from build123d import *

# Parameters (mm, degrees)
SALIENTE_EXTRUIR1_DEPTH = 25
REDONDEO1_R             = 7
VACIADO1_T              = -3


with BuildPart() as part:
    # Croquis1 → Saliente-Extruir1 (new body)
    with BuildSketch(Plane.XY):
        with BuildLine():
            Line((-110, 65.5), (110, 65.5))
            ThreePointArc((110, 65.5), (122.727922061, 60.227922061), (128, 47.5))
            Line((128, 47.5), (128, -47.5))
            ThreePointArc((128, -47.5), (122.727922061, -60.227922061), (110, -65.5))
            Line((110, -65.5), (-110, -65.5))
            ThreePointArc((-110, -65.5), (-122.727922061, -60.227922061), (-128, -47.5))
            Line((-128, -47.5), (-128, 47.5))
            ThreePointArc((-128, 47.5), (-122.727922061, 60.227922061), (-110, 65.5))
        make_face()
    extrude(amount=SALIENTE_EXTRUIR1_DEPTH)

    # Redondeo1
    redondeo1_edges = [part.edges().sort_by_distance(p)[0] for p in [
        (-122.727922061, 60.227922061, 25),
        (-128, 0, 25),
        (-122.727922061, -60.227922061, 25),
        (0, -65.5, 25),
        (122.727922061, -60.227922061, 25),
        (128, 0, 25),
        (122.727922061, 60.227922061, 25),
        (0, 65.5, 25),
    ]]
    fillet(redondeo1_edges, radius=REDONDEO1_R)

    # Vaciado1
    vaciado1_openings = [part.faces().sort_by_distance(p)[0] for p in [
        (0, 0, 0),
    ]]
    offset(amount=VACIADO1_T, openings=vaciado1_openings, kind=Kind.INTERSECTION)


solid = part.part
Design review of the part built by this model. Coordinates are the model's own, in mm. A direction names the side the tool comes from. Coordinates: 2 decimals unless noted, no trailing zeros. Order: outer loops, then holes, each group sorted by start corner. A loop starts at its lowest first (then second) coordinate and runs counter-clockwise, first axis right, second up. Notation, with made-up numbers: (27.5, 18.5) -> (38.5, 18.5) arc R26 cw to (38.5, 38.5) -> close; hole circle Ø3 at (28, 18). An arc over 180 degrees is marked (long way). One line per item, written item: value.
1) To check wall thickness, follow probe 1 along Y at (x, z) = (82, 11.5); probe 2 along X at (y, z) = (-46, 4.75); probe 3 along Z at (x, y) = (-69, -10). State the ranges of each line that lie inside material, in increasing order. Write a range as [from, to].
Output values:
probe 1: y = [-65.5, -62.5], [62.5, 65.5]
probe 2: x = [-128, -125], [125, 128]
probe 3: z = [22, 25]
2) Machinability: for faces 4 (the face through (-120.49, -58.22, 8.87)), 5 (the face through (122.587, 60.367, 8.874)), which of the approach directions +Z, -Z, +X, -X, +Y, -Y give a long, thin tool a straight path to every point of the face, cutting with its end or side? Answer none if there is none.
Output values:
face 4: -Z
face 5: +Z, -Z, +X, +Y
3) Draft analysis for pull direction Y (two halves, no side actions). For faces 1 (the face through (-126, 0.7, 22.9)), 2 (the face through (125, 1, 9)), 3 (the face through (-122.587, -60.367, 8.874)), state which applies: +Y half, -Y half, draft (parallel to the pull), parting line (faces both ways), or undercut.
Output values:
face 1: draft
face 2: undercut
face 3: -Y half
4) We need section C-C, the plane x = 61.5. Give the boundary of the cut face in (y, z), then the cut area to 3 significant figures.
Output values:
outline: (-65.5, 0) -> (-62.5, 0) -> (-62.5, 18) arc R4 cw to (-58.5, 22) -> (58.5, 22) arc R4 cw to (62.5, 18) -> (62.5, 0) -> (65.5, 0) -> (65.5, 18) arc R7 ccw to (58.5, 25) -> (-58.5, 25) arc R7 ccw to (-65.5, 18) -> close
area: 511 mm2
5) We need section A-A, the plane z = 2.75. Give the boundary of the cut face in (x, y), then the cut area to 3 significant figures.
Output values:
outline: (-128, -47.5) arc R18 ccw to (-110, -65.5) -> (110, -65.5) arc R18 ccw to (128, -47.5) -> (128, 47.5) arc R18 ccw to (110, 65.5) -> (-110, 65.5) arc R18 ccw to (-128, 47.5) -> close; hole (-125, -47.5) arc R15 ccw to (-110, -62.5) -> (110, -62.5) arc R15 ccw to (125, -47.5) -> (125, 47.5) arc R15 ccw to (110, 62.5) -> (-110, 62.5) arc R15 ccw to (-125, 47.5) -> close
area: 2,200 mm2
6) Clearance check with a flat-ended pin moving along its axis: P1, Ø4, axis at x = 51, y = -3.5, coming from the -Z side. State where the tip first meets the part, or that it passes through.
Output values:
P1: stops at z = 22
7) We need section B-B, the plane y = 43. Give the boundary of the cut face in (x, z), then the cut area to 3 significant figures.
Output values:
outline: (-128, 0) -> (-125, 0) -> (-125, 18) arc R4 cw to (-121, 22) -> (121, 22) arc R4 cw to (125, 18) -> (125, 0) -> (128, 0) -> (128, 18) arc R7 ccw to (121, 25) -> (-121, 25) arc R7 ccw to (-128, 18) -> close
area: 886 mm2
